from build123d import *

# Parameters (mm, degrees)
SKETCH_1_W              = 18
SKETCH_1_H              = 18
EXTRUDE_2_DEPTH         = 10
EXTRUDE_3_DEPTH         = 90
CUT_EXTRUDE_3_DEPTH     = 86
CUT_EXTRUDE_START       = -100
CUT_EXTRUDE_5_OUTLINE_R = 5.5
CUT_EXTRUDE_5_DEPTH     = 93
SKETCH_7_R              = 8
CUT_EXTRUDE_6_DEPTH     = 7
FILLET_6_R              = 3
FILLET_7_R              = 3
FILLET_8_R              = 3
FILLET_9_R              = 3


# Read off the part's stored shape, not the designer's step: 切除-拉伸5
with BuildPart() as part:
    # 草图1 → 凸台-拉伸2 (new body)
    with BuildSketch(Plane.XY):
        with Locations((-9, -9)):
            Rectangle(SKETCH_1_W, SKETCH_1_H)
    extrude(amount=-EXTRUDE_2_DEPTH)

    # Sketch 3D_1 → 凸台-拉伸3 (add)
    with BuildSketch(Plane(origin=(9.495592889, -27.495592889, -10), x_dir=(-0.7071067811865476, 0.7071067811865476, -9.817405728081993e-13), z_dir=(-1.3883908327972863e-12, 0, 1.0))):
        Polygon((0, 0), (26.156718308, 26.156718308), (52.313436617, 0), (26.156718308, -26.156718308), align=None)
    extrude(amount=-EXTRUDE_3_DEPTH)

    # 草图6 → 切除-拉伸3 (cut)
    with BuildSketch(Plane(origin=(0, 0, -100), x_dir=(-1.0, 0, -1.3537169902663766e-12), z_dir=(1.3537169902663766e-12, -3.467772761410138e-14, -1.0))):
        with BuildLine():
            ThreePointArc((20.610593598, -20.610593598), (1.033022784, 5.357543015), (12.708084345, -24.995683102))
            ThreePointArc((12.708084345, -24.995683102), (15.102764846, -21.155695433), (11.262777177, -18.761014932))
            ThreePointArc((11.262777177, -18.761014932), (4.138326818, -0.238624142), (16.085110199, -16.085110199))
            ThreePointArc((16.085110199, -16.085110199), (16.085110199, -20.610593598), (20.610593598, -20.610593598))
        make_face()
    extrude(amount=-CUT_EXTRUDE_3_DEPTH, mode=Mode.SUBTRACT)

    # 切除-拉伸5 outline → 切除-拉伸5 (cut)
    with BuildSketch(Plane.XY.offset(CUT_EXTRUDE_START)):
        with Locations((-9, -9)):
            Circle(CUT_EXTRUDE_5_OUTLINE_R)
    extrude(amount=CUT_EXTRUDE_5_DEPTH, mode=Mode.SUBTRACT)

    # 草图7 → 切除-拉伸6 (cut)
    with BuildSketch(Plane.XY):
        with Locations((-9, -9)):
            Circle(SKETCH_7_R)
    extrude(amount=-CUT_EXTRUDE_6_DEPTH, mode=Mode.SUBTRACT)

    # 圆角6
    fillet_6_edges = [part.edges().sort_by_distance(p)[0] for p in [
        (-18, 0, -5),
    ]]
    fillet(fillet_6_edges, radius=FILLET_6_R)

    # 圆角7
    fillet_7_edges = [part.edges().sort_by_distance(p)[0] for p in [
        (-18, -18, -5),
    ]]
    fillet(fillet_7_edges, radius=FILLET_7_R)

    # 圆角8
    fillet_8_edges = [part.edges().sort_by_distance(p)[0] for p in [
        (0, 0, -5),
    ]]
    fillet(fillet_8_edges, radius=FILLET_8_R)

    # 圆角9
    fillet_9_edges = [part.edges().sort_by_distance(p)[0] for p in [
        (0, -18, -5),
    ]]
    fillet(fillet_9_edges, radius=FILLET_9_R)


solid = part.part
Could you check a few things on this model? Use its own coordinates, in mm. A direction names the side the tool comes from. Round coordinates to 2 decimals unless told otherwise and drop trailing zeros. Order: outer loops, then holes, each group sorted by start corner. A loop starts at its lowest first (then second) coordinate and runs counter-clockwise, first axis right, second up.
(1) Which directions (+Z, -Z, +X, -X, +Y, -Y) give clear straight access to the entire face, cutting with the end or side of a thin tool? Please do faces 1 (the flat face through (-16, -1, -14)), 2 (the flat face through (-9, 0, -5)), 3 (the cylindrical face through (-17.14, -0.9, -5.07)), 4 (the flat face through (-7.3, -3.6, -7)).
Response values:
face 1: -Z
face 2: +Z, +X, -X, +Y
face 3: +Z, -X, +Y
face 4: +Z
(2) Imagine slicing it at C-C (z = -37). Write out the boundary of the cut face in (x, y).
Response values:
outline: (-27.5, -27.5) - (9.5, -27.5) - (9.5, 9.5) - (-27.5, 9.5) - close; hole (-20.61, -20.61) arc R3.2 ccw to (-16.09, -16.09) arc R10.02 cw (long way) to (-11.26, -18.76) arc R3.2 ccw to (-12.71, -25) arc R16.42 ccw (long way) to start; hole circle Ø11 at (-9, -9)
(3) Imagine slicing it at D-D (x = -23). Write out the boundary of the cut face in (y, z).
Response values:
outline: (-27.5, -100) - (-17.58, -100) - (-17.58, -14) - (-0.42, -14) - (-0.42, -100) - (9.5, -100) - (9.5, -10) - (-27.5, -10) - close
(4) Imagine slicing it at A-A (y = -9). Write out the boundary of the cut face in (x, z), plus the area to 3 significant figures.
Response values:
outline: (-27.5, -100) - (-25.42, -100) - (-25.42, -14) - (-19.02, -14) - (-19.02, -100) - (-14.5, -100) - (-14.5, -7) - (-17, -7) - (-17, 0) - (-18, 0) - (-18, -10) - (-27.5, -10) - close; (-3.5, -100) - (1.02, -100) - (1.02, -14) - (7.42, -14) - (7.42, -100) - (9.5, -100) - (9.5, -10) - (0, -10) - (0, 0) - (-1, 0) - (-1, -7) - (-3.5, -7) - close
area: 1,270 mm2
(5) Please list where these lines run through material, in increasing order: line 1 along Y through (x, z) = (-9, -63.5); line 2 along Y through (x, z) = (-7.5, -18.5); line 3 along X through (y, z) = (-12.5, -25.5).
Response values:
line 1: y = -27.5 to -25.42, -19.02 to -14.5, -3.5 to 1.02, 7.42 to 9.5
line 2: y = -27.5 to -25.35, -18.91 to -14.29, -3.71 to 0.91, 7.35 to 9.5
line 3: x = -27.5 to -25.04, -18.39 to -13.24, -4.76 to 0.39, 7.04 to 9.5
(6) If we mould it in two halves opening along X, with no side actions, what happens to faces 5 (the flat face through (-18, -9, -5)), 6 (the cylindrical face through (-1.615, 5.665, -57.602)), 7 (the flat face through (-9, 9.496, -54))? For each: released by +X, released by -X, zero draft, split by the parting line, or undercut.
Response values:
face 5: released by -X
face 6: undercut
face 7: zero draft
(7) I'm going to push flat-ended pins straight in: pin 1 (5 mm diameter, centred on x = -2.5, y = 4, fed in from -Z); pin 2 (3 mm diameter, centred on x = -8.5, z = -3, fed in from +Y); pin 3 (3 mm diameter, centred on x = -8.5, z = -4, fed in from -Y); pin 4 (5 mm diameter, centred on y = -11, z = -5.5, fed in from +X). Where does each tip first touch, or does it pass through?
Response values:
pin 1: stops at z = -100
pin 2: stops at y = 0
pin 3: stops at y = -18
pin 4: stops at x = 0
